Study the drawing (mm; zero at the part's minimum x, y, z) and answer. Give positions to 0.01 mm unless a question says otherwise; leave off trailing zeros. Write each loop counter-clockwise with the first axis right and the second up, starting at its lowest first coordinate (ties: lowest second). Pieces come first, ordered by that corner, then holes. Notation, with made-up numbers: M -33.5,76.5 L -25.5,76.5 A24 cw -25.5,95.5 Z; hole C 20.25,15.5 d2. An arc over 180 degrees is marked long. Use a Markdown table: item, result. Add a question column.
Item 1: A cutting plane is placed at D-D on x = 12. Determine the outline of the cut face in (y, z).
Item 2: Given P1, Ø1.5, axis at y = 2, z = 68, coming from the +X side; P2, Ø0.9, axis at x = 11, y = 2, coming from the +Z side; P3, Ø0.9, axis at x = 74.5, y = 1.5, coming from the -Z side, each flat-ended and moving along its own axis, determine where each tip first touches the part or whether it passes through.
Item 3: A cutting plane is placed at A-A on y = 2.2. Determine the outline of the cut face in (x, z), then the cut area to 3 significant figures.
Item 4: A cutting plane is placed at B-B on x = 43.5. Determine the outline of the cut face in (y, z), then the cut area to 3 significant figures.
Item 5: A cutting plane is placed at C-C on z = 69.5. Determine the outline of the cut face in (x, y), then the cut area to 3 significant figures.
Item 6: Consider probe 1 along Z at (x, y) = (41.5, 2.35); probe 2 along Z at (x, y) = (71, 1.45). Determine where each line is inside the solid, lowest interval first. Write a range as [from, to].
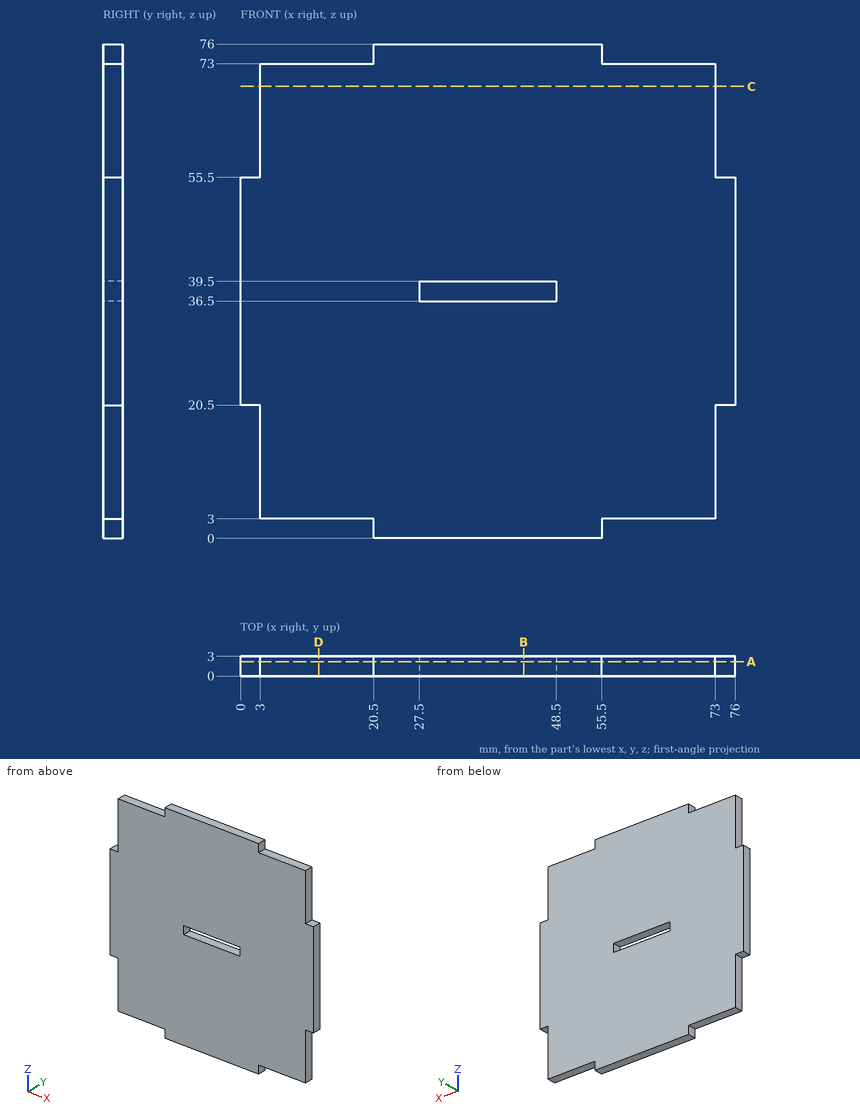
Filled in:
| question | item | result |
|---|---|---|
| 1 | outline | M 0,3 L 3,3 L 3,73 L 0,73 Z |
| 2 | P1 | x = 73 |
| 2 | P2 | z = 73 |
| 2 | P3 | z = 20.5 |
| 3 | outline | M 0,20.5 L 3,20.5 L 3,3 L 20.5,3 L 20.5,0 L 55.5,0 L 55.5,3 L 73,3 L 73,20.5 L 76,20.5 L 76,55.5 L 73,55.5 L 73,73 L 55.5,73 L 55.5,76 L 20.5,76 L 20.5,73 L 3,73 L 3,55.5 L 0,55.5 Z; hole M 27.5,36.5 L 48.5,36.5 L 48.5,39.5 L 27.5,39.5 Z |
| 3 | area | 5,260 mm² |
| 4 | outline | M 0,0 L 3,0 L 3,36.5 L 0,36.5 Z; M 0,39.5 L 3,39.5 L 3,76 L 0,76 Z |
| 4 | area | 219 mm² |
| 5 | outline | M 3,0 L 73,0 L 73,3 L 3,3 Z |
| 5 | area | 210 mm² |
| 6 | probe 1 | [0, 36.5], [39.5, 76] |
| 6 | probe 2 | [3, 73] |
